Design review of the part built by this model. Coordinates are the model's own, in mm. Face numbers are marked on the shaded views. A direction names the side the tool comes from. Round coordinates to 2 decimals unless told otherwise and drop trailing zeros. Order: outer loops, then holes, each group sorted by start corner. A loop starts at its lowest first (then second) coordinate and runs counter-clockwise, first axis right, second up. Notation, with made-up numbers: (-31, 43) - (28, 43) arc R8 ccw to (28, 54) - close; hole circle Ø4 at (-40, 44.25). An arc over 180 degrees is marked (long way). Write item = value, one per line.
from build123d import *

# Parameters (mm, degrees)
F0_R     = 11.5
F0_R_2   = 8.5
F1_DEPTH = 4
F2_DEPTH = 20
F4_DEPTH = 10


# Not quite as in the source:
# - a feature names something its author has since deleted; it is built from what else it names


with BuildPart() as f1:
    # F0 (on Top) → F1 (new body)
    with BuildSketch(Plane.XY):
        Polygon((-43.75, -9.9592921435), (-26.5, 0), (-43.75, 9.9592921435), align=None)
        Polygon((-32.5, 0), (-40.75, -4.7631397208), (-40.75, 4.7631397208), align=None, mode=Mode.SUBTRACT)
        with BuildLine():
            Line((-43.75, 9.9592921435), (-26.5, 0))
            ThreePointArc((-26.5, 0), (-22.1457987188, 14.5538173379), (-10.514067992, 24.324974291))
            Line((-10.514067992, 24.324974291), (-43.75, 9.9592921435))
        make_face()
        with BuildLine():
            ThreePointArc((-10.514067992, 24.324974291), (-22.1457987188, 14.5538173379), (-26.5, 0))
            ThreePointArc((-26.5, 0), (-22.1457987188, -14.5538173379), (-10.514067992, -24.324974291))
            ThreePointArc((-10.514067992, -24.324974291), (14.5538173379, -22.1457987188), (26.5, 0))
            ThreePointArc((26.5, 0), (14.5538173379, 22.1457987188), (-10.514067992, 24.324974291))
        make_face()
        Circle(F0_R, mode=Mode.SUBTRACT)
        Circle(F0_R)
        Circle(F0_R_2, mode=Mode.SUBTRACT)
        with BuildLine():
            ThreePointArc((-10.514067992, -24.324974291), (-22.1457987188, -14.5538173379), (-26.5, 0))
            Line((-26.5, 0), (-43.75, -9.9592921435))
            Line((-43.75, -9.9592921435), (-10.514067992, -24.324974291))
        make_face()
    extrude(amount=-F1_DEPTH)

    # F0 (on Top) → F2 (join)
    with BuildSketch(Plane.XY):
        Polygon((-43.75, -9.9592921435), (-26.5, 0), (-43.75, 9.9592921435), align=None)
        Polygon((-32.5, 0), (-40.75, -4.7631397208), (-40.75, 4.7631397208), align=None, mode=Mode.SUBTRACT)
        Circle(F0_R)
        Circle(F0_R_2, mode=Mode.SUBTRACT)
    extrude(amount=F2_DEPTH)

    # F3 (on face) → F4 (cut)
    with BuildSketch(Plane(origin=(-43.75, 0, 0), x_dir=(0, -1, 0), z_dir=(-1, 0, 0))):
        Polygon((-9.9592921435, 1.25), (-9.9592921435, 0), (-8.7092921435, 0), align=None)
        Polygon((-9.9592921435, 3.75), (-9.9592921435, 1.25), (-8.7092921435, 2.5), align=None)
        Polygon((-8.7092921435, 5), (-9.9592921435, 6.25), (-9.9592921435, 3.75), align=None)
        Polygon((-8.7092921435, 7.5), (-9.9592921435, 8.75), (-9.9592921435, 6.25), align=None)
        Polygon((-8.7092921435, 10), (-9.9592921435, 11.25), (-9.9592921435, 8.75), align=None)
        Polygon((-8.7092921435, 12.5), (-9.9592921435, 13.75), (-9.9592921435, 11.25), align=None)
        Polygon((-8.7092921435, 15), (-9.9592921435, 16.25), (-9.9592921435, 13.75), align=None)
        Polygon((-8.7092921435, 17.5), (-9.9592921435, 18.75), (-9.9592921435, 16.25), align=None)
        Polygon((-9.9592921435, 18.75), (-8.7092921435, 20), (-9.9592921435, 20), align=None)
    extrude(amount=-F4_DEPTH, mode=Mode.SUBTRACT)


solid = f1.part
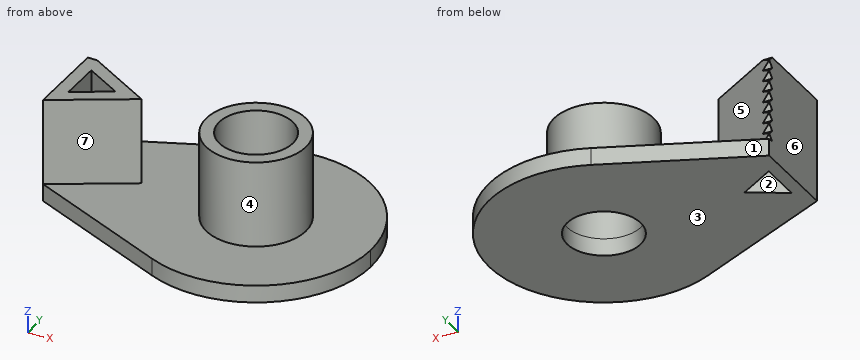
1) To check wall thickness, follow L1, parallel to Y at x = 0, z = 13.25; L2, parallel to X at y = 5, z = 5.25; L3, parallel to Z at x = -14.5, y = 21. State the ranges of each line that lie inside material, in increasing order. Write a range as from..to.
Findings:
L1 = -11.5..-8.5, 8.5..11.5
L2 = -43.75..-35.16, -10.36..-6.87, 6.87..10.36
L3 = -4..0
2) The part is to be moulded in two halves that separate along X. For the marked faces 1, 2 and 3, say which applies: released by +X, released by -X, zero draft, split by the parting line, or undercut.
Findings:
face_1 = released by -X
face_2 = undercut
face_3 = zero draft
3) For the marked faces 4, 5, 6 and 7, list the 3-axis set-ups (+Z, -Z, +X, -X, +Y, -Y) from which the entire face can be reached by the end or side of a thin tool; tool diameter is ignored.
Findings:
face_4 = +Z
face_5 = +Z, +Y
face_6 = +Z, -Z, -X, +Y, -Y
face_7 = +Z, -Y
4) We need section C-C on x = 21. Write out the cut boundary in (y, z).
Findings:
outline = (-16.16, -4) - (16.16, -4) - (16.16, 0) - (-16.16, 0) - close
5) We need section B-B on y = -19.5. Write out the cut boundary in (x, z).
Findings:
outline = (-21.68, -4) - (17.94, -4) - (17.94, 0) - (-21.68, 0) - close
6) We need section A-A on x = 0. Write out the cut boundary in (y, z), and give its area (3 significant figures).
Findings:
outline = (-26.5, -4) - (-8.5, -4) - (-8.5, 20) - (-11.5, 20) - (-11.5, 0) - (-26.5, 0) - close; (8.5, -4) - (26.5, -4) - (26.5, 0) - (11.5, 0) - (11.5, 20) - (8.5, 20) - close
area = 264 mm^2
7) Clearance check with flat-ended pins moving along their axes: pin 1 Ø5 at (x, y) = (-35, -11) entering from +Z; pin 2 Ø10 at (x, z) = (13, 17) entering from +Y; pin 3 Ø10 at (y, z) = (-7.5, 11.5) entering from +X (3 decimals); pin 4 Ø8 at (y, z) = (-11.5, 8.5) entering from -X. State where each tip first meets the part, or that it passes through.
Findings:
pin_1 = 0
pin_2 = 8.26
pin_3 = 11.225
pin_4 = -43.75
